from build123d import *

# Parameters (mm, degrees)
SKETCH_1_W          = 25
SKETCH_1_H          = 30
EXTRUDE_1_DEPTH     = 10
SKETCH_2_W          = 20.5
SKETCH_2_H          = 30
CUT_EXTRUDE_1_DEPTH = 3
SKETCH_3_R          = 1.25
CUT_EXTRUDE_2_DEPTH = 12
SKETCH_5_W          = 10
SKETCH_5_H          = 10
CUT_EXTRUDE_4_DEPTH = 12
FILLET_1_R          = 3
EXTRUDE_2_DEPTH     = 3
FILLET_2_R          = 5
SKETCH_7_R          = 1.75
CUT_EXTRUDE_5_DEPTH = 3


with BuildPart() as part:
    # 스케치1 → 보스-돌출1 (new body)
    with BuildSketch(Plane.XY):
        with Locations((12.5, 15)):
            Rectangle(SKETCH_1_W, SKETCH_1_H)
    extrude(amount=EXTRUDE_1_DEPTH)

    # 스케치2 → 컷-돌출1 (cut)
    with BuildSketch(Plane.XY.offset(10)):
        with Locations((12.5, 15)):
            Rectangle(SKETCH_2_W, SKETCH_2_H)
    extrude(amount=-CUT_EXTRUDE_1_DEPTH, mode=Mode.SUBTRACT)

    # 스케치3 → 컷-돌출2 (cut)
    with BuildSketch(Plane(origin=(0, 30, 0), x_dir=(1, 0, 0), z_dir=(0, 1, 0))):
        with Locations(Location((7.5, -3.5, 0), (0, 0, 270))):
            Circle(SKETCH_3_R)
        with Locations(Location((17.5, -3.5, 0), (0, 0, 270))):
            Circle(SKETCH_3_R)
    extrude(amount=-CUT_EXTRUDE_2_DEPTH, mode=Mode.SUBTRACT)

    # 스케치5 → 컷-돌출4 (cut)
    with BuildSketch(Plane(origin=(0, 0, 0), x_dir=(-1, 0, 0), z_dir=(0, 0, -1))):
        with Locations((-12.5, 5)):
            Rectangle(SKETCH_5_W, SKETCH_5_H)
    extrude(amount=-CUT_EXTRUDE_4_DEPTH, mode=Mode.SUBTRACT)

    # 필렛1
    fillet_1_edges = [part.edges().sort_by_distance(p)[0] for p in [
        (17.5, 10, 3.5),
        (7.5, 10, 3.5),
        (25, 15, 0),
        (0, 15, 0),
    ]]
    fillet(fillet_1_edges, radius=FILLET_1_R)

    # 스케치6 → 보스-돌출2 (add)
    with BuildSketch(Plane.XZ):
        Polygon((22.75, 10), (37.5, 10), (37.5, -10), (17.5, -10), (17.5, 7), (22.75, 7), align=None)
        with BuildLine():
            Line((7.5, -10), (7.5, 0))
            Line((7.5, 0), (3, 0))
            ThreePointArc((3, 0), (0.878679656, 0.878679656), (0, 3))
            Line((0, 3), (0, 10))
            Line((0, 10), (-12.5, 10))
            Line((-12.5, 10), (-12.5, -10))
            Line((-12.5, -10), (-3.976787784, -10))
            Line((-3.976787784, -10), (7.5, -10))
        make_face()
    extrude(amount=-EXTRUDE_2_DEPTH)

    # 필렛2
    fillet_2_edges = [part.edges().sort_by_distance(p)[0] for p in [
        (-12.5, 1.5, -10),
        (37.5, 1.5, -10),
    ]]
    fillet(fillet_2_edges, radius=FILLET_2_R)

    # 스케치7 → 컷-돌출5 (cut)
    with BuildSketch(Plane(origin=(0, 3, 0), x_dir=(1, 0, 0), z_dir=(0, 1, 0))):
        with Locations(Location((32.5, 5, 0), (0, 0, 270))):
            Circle(SKETCH_7_R)
        with Locations(Location((-7.5, 5, 0), (0, 0, 270))):
            Circle(SKETCH_7_R)
    extrude(amount=-CUT_EXTRUDE_5_DEPTH, mode=Mode.SUBTRACT)


solid = part.part
Can you work these out from the model? Positions are in its coordinate system, mm. A direction names the side the tool comes from. Coordinates: 2 decimals unless noted, no trailing zeros. Order: outer loops, then holes, each group sorted by start corner. A loop starts at its lowest first (then second) coordinate and runs counter-clockwise, first axis right, second up. Notation, with made-up numbers: (62, 11) - (82, 11) arc R28 cw to (82, 30) - close; hole circle Ø7 at (23, 43). An arc over 180 degrees is marked (long way). Answer as a JSON object with one key per item and string values. Group by question number.
Q1. On a 3-axis mill with a long thin cutter (end or side, diameter ignored), from which of +Z, -Z, +X, -X, +Y, -Y can I reach the whole of each face in a straight line? I mean faces 5 (the face through (0.86, 16.69, 0.9)), 6 (the face through (8.36, 9.1, 3.55)), 7 (the face through (12, 19, 7)), 8 (the face through (8, 18, 3)). Say none if no direction works.
Q2. We'd pull the mould along X, two halves only. Please class faces 1 (the face through (13, 10, 3)), 2 (the face through (37.5, 1, 3)), 3 (the face through (0, 16, 6)), 4 (the face through (-3, 0, 0)): +X half, -X half, draft (parallel to the pull), parting line (faces both ways), or undercut.
Q3. Imagine slicing it at A-A (z = -1.5). Please give me the cut outline in (x, y), and give its area (3 significant figures).
Q4. Imagine slicing it at D-D (z = 3.5). Please give me the cut outline in (x, y).
Q5. Imagine slicing it at B-B (y = 25.25). Please give me the cut outline in (x, z), and give its area (3 significant figures).
Q6. I need wall thicknesses on line 1 (X direction, y = 0.75, z = -5); line 2 (X direction, y = 23.5, z = 3.5); line 3 (X direction, y = 22, z = 8.25). Which ranges of each line are inside material? Lowest first, please. Write a range as from..to.
Q7. Will these pins go through, and if not, where does the flat tip stop? P1, Ø6, axis at x = -2, y = 19.5, coming from the -Z side; P2, Ø5.5, axis at y = 11, z = 7.5, coming from the +X side; P3, Ø1.5, axis at y = 4.5, z = 3.5, coming from the -X side; P4, Ø1.5, axis at x = 27, y = 16.5, coming from the +Z side.
Q8. Imagine slicing it at C-C (y = 11.75). Please give me the cut outline in (x, z), and give its area (3 significant figures).
Determined:
{
 "1": {"face 5": "-Z, -X, +Y", "face 6": "+Z, -Z, -Y", "face 7": "+Z, +Y, -Y", "face 8": "+Y"},
 "2": {"face 1": "undercut", "face 2": "+X half", "face 3": "-X half", "face 4": "draft"},
 "3": {"outline": "(-12.5, 0) - (7.5, 0) - (7.5, 3) - (-12.5, 3) - close; (17.5, 0) - (37.5, 0) - (37.5, 3) - (17.5, 3) - close", "area": "120 mm2"},
 "4": {"outline": "(-12.5, 0) - (7.5, 0) - (7.5, 7) arc R3 cw to (10.5, 10) - (14.5, 10) arc R3 cw to (17.5, 7) - (17.5, 0) - (37.5, 0) - (37.5, 3) - (25, 3) - (25, 30) - (18.75, 30) - (18.75, 18) - (16.25, 18) - (16.25, 30) - (8.75, 30) - (8.75, 18) - (6.25, 18) - (6.25, 30) - (0, 30) - (0, 3) - (-12.5, 3) - close"},
 "5": {"outline": "(0, 3) arc R3 ccw to (3, 0) - (22, 0) arc R3 ccw to (25, 3) - (25, 10) - (22.75, 10) - (22.75, 7) - (2.25, 7) - (2.25, 10) - (0, 10) - close; hole circle Ø2.5 at (7.5, 3.5); hole circle Ø2.5 at (17.5, 3.5)", "area": "175 mm2"},
 "6": {"line 1": "x = -12.5..-9.25, -5.75..7.5, 17.5..30.75, 34.25..37.5", "line 2": "x = 0..6.25, 8.75..16.25, 18.75..25", "line 3": "x = 0..2.25, 22.75..25"},
 "7": {"P1": "stops at z = 0.76", "P2": "stops at x = 25", "P3": "stops at x = 0", "P4": "passes through"},
 "8": {"outline": "(0, 3) arc R3 ccw to (3, 0) - (22, 0) arc R3 ccw to (25, 3) - (25, 10) - (22.75, 10) - (22.75, 7) - (2.25, 7) - (2.25, 10) - (0, 10) - close", "area": "185 mm2"}
}
